from build123d import *

# Parameters (mm, degrees)
SKETCH1_W           = 240
SKETCH1_H           = 38
BOSS_EXTRUDE1_DEPTH = 3
SKETCH2_W           = 38
SKETCH2_H           = 18
CUT_EXTRUDE1_DEPTH  = 3
FILLET1_R           = 5


with BuildPart() as part:
    # Sketch1 → Boss-Extrude1 (new body)
    with BuildSketch(Plane(origin=(0, 0, 0), x_dir=(1, 0, 0), z_dir=(0, 1, 0))):
        Rectangle(SKETCH1_W, SKETCH1_H)
    extrude(amount=BOSS_EXTRUDE1_DEPTH)

    # Sketch2 → Cut-Extrude1 (cut)
    with BuildSketch(Plane(origin=(0, 3, 0), x_dir=(1, 0, 0), z_dir=(0, 1, 0))):
        with Locations((-101, -10)):
            Rectangle(SKETCH2_W, SKETCH2_H)
        with Locations((101, -10)):
            Rectangle(SKETCH2_W, SKETCH2_H)
    extrude(amount=-CUT_EXTRUDE1_DEPTH, mode=Mode.SUBTRACT)

    # Fillet1
    fillet1_edges = [part.edges().sort_by_distance(p)[0] for p in [
        (-82, 1.5, 1),
        (82, 1.5, 1),
    ]]
    fillet(fillet1_edges, radius=FILLET1_R)


solid = part.part
The listing builds one solid part. Answer for the finished solid, in the listing's coordinates (mm). Round coordinates to 2 decimals unless told otherwise and drop trailing zeros. Order: outer loops, then holes, each group sorted by start corner. A loop starts at its lowest first (then second) coordinate and runs counter-clockwise, first axis right, second up. Notation, with made-up numbers: (82, 43) - (96, 43) arc R18 ccw to (96, 74) - close; hole circle Ø4 at (-14.5, -12.75). An arc over 180 degrees is marked (long way). Write item = value, one per line. Start each with the question number.
1) Section A-A, the plane y = 1.2 is taken. Write down the section's boundary in (x, z), plus the area to 3 significant figures.
2) Straight lines are drawn through the part: L1, parallel to Z at x = 91, y = 0.55; L2, parallel to X at y = 2, z = 12; L3, parallel to X at y = 2.1, z = 4.5. For each, find the intervals that lie inside material, in ascending order.
3) Section C-C, the plane z = 11 is taken. Write down the section's boundary in (x, y).
4) Section B-B, the plane x = 95.5 is taken. Write down the section's boundary in (y, z), plus the area to 3 significant figures.
5) Given pin 1 (1.5 mm diameter, centred on y = 2, z = 12.5, fed in from -X), flat-ended and moving along its own axis, determine where the tip first touches the part or whether it passes through.
Results list:
q1.outline = (-120, -19) - (120, -19) - (120, 1) - (87, 1) arc R5 cw to (82, 6) - (82, 19) - (-82, 19) - (-82, 6) arc R5 cw to (-87, 1) - (-120, 1) - close
q1.area = 7,760 mm^2
q2.L1 = -19 to 1
q2.L2 = -82 to 82
q2.L3 = -82.23 to 82.23
q3.outline = (-82, 0) - (82, 0) - (82, 3) - (-82, 3) - close
q4.outline = (0, -19) - (3, -19) - (3, 1) - (0, 1) - close
q4.area = 60.0 mm^2
q5.pin_1 = -82
